For this review, take the finished solid that the model builds, in its own axes (mm). Coordinates: 2 decimals unless noted, no trailing zeros. Write each loop counter-clockwise with the first axis right and the second up, starting at its lowest first coordinate (ties: lowest second). Pieces come first, ordered by that corner, then holes. Notation, with made-up numbers: M 55,36 L 66,36 A16 ccw 66,46 Z; hole C 47.5,54 d4. An arc over 180 degrees is marked long. One line per question, with ' | ' between items.
from build123d import *

# Parameters (mm, degrees)
F0_W     = 240
F0_H     = 55.88
F1_DEPTH = 5


with BuildPart() as f1:
    # F0 (on Top) → F1 (new body)
    with BuildSketch(Plane.XY):
        with Locations((-1.303092, 10.622495)):
            Rectangle(F0_W, F0_H)
        Polygon((-77.501602, 1.566828), (-77.501602, 18.42894), (-73.263034, 18.42894), (-73.263034, 5.436821), (-66.813052, 5.436821), (-66.813052, 1.566828), align=None, mode=Mode.SUBTRACT)
        Polygon((-65.523051, 1.566828), (-65.523051, 18.42894), (-53.171746, 18.42894), (-53.171746, 14.558948), (-61.376628, 14.558948), (-61.376628, 11.610381), (-53.63664, 11.610381), (-53.63664, 8.016816), (-61.284486, 8.016816), (-61.284486, 5.436821), (-52.623071, 5.436821), (-52.623071, 1.566828), align=None, mode=Mode.SUBTRACT)
        Polygon((-46.633799, 1.566828), (-52.623071, 18.42894), (-48.753079, 18.42894), (-44.975229, 7.187532), (-40.736664, 18.42894), (-36.682386, 18.42894), (-43.408804, 1.566828), align=None, mode=Mode.SUBTRACT)
        Polygon((-36.069706, 1.566828), (-36.069706, 18.42894), (-23.595029, 18.42894), (-23.595029, 14.341751), (-32.273065, 14.341751), (-32.273065, 11.978536), (-24.56356, 11.978536), (-24.56356, 7.833225), (-31.885654, 7.833225), (-31.885654, 5.436821), (-23.517547, 5.436821), (-23.517547, 1.566828), align=None, mode=Mode.SUBTRACT)
        Polygon((-22.122035, 1.566828), (-22.122035, 18.42894), (-16.931558, 18.42894), (-16.931558, 5.461609), (-10.812703, 5.461609), (-10.812703, 1.566828), align=None, mode=Mode.SUBTRACT)
        with BuildLine():
            Line((0, 1.486314), (0, 5.613023))
            ThreePointArc((0, 5.613023), (-1.939251, 14.918573), (-3.923162, 5.622442))
            Line((-3.923162, 5.622442), (-3.923162, 1.491197))
            ThreePointArc((-3.923162, 1.491197), (-1.939969, 18.855408), (0, 1.486314))
        make_face(mode=Mode.SUBTRACT)
        Polygon((12.757826, 1.425337), (7.98934, 1.425337), (7.98934, 18.42894), (12.757826, 18.42894), (19.847259, 7.966181), (19.847259, 18.42894), (23.944732, 18.348456), (23.944732, 1.425337), (19.847259, 1.425337), (12.757826, 11.888096), align=None, mode=Mode.SUBTRACT)
        Polygon((26.369521, 1.566828), (26.369521, 18.42894), (38.351353, 18.42894), (38.351353, 14.247308), (30.56819, 14.247308), (30.56819, 12.04724), (38.016446, 12.04724), (38.016446, 7.966181), (30.505024, 7.966181), (30.505024, 5.552883), (39.282415, 5.552883), (39.282415, 1.566828), align=None, mode=Mode.SUBTRACT)
        Polygon((39.282415, 14.247308), (39.282415, 18.42894), (52.912835, 18.42894), (52.912835, 14.247308), (48.958834, 14.247308), (48.958834, 1.566828), (43.528017, 1.566828), (43.528017, 14.247308), align=None, mode=Mode.SUBTRACT)
        Polygon((54.121282, 1.566828), (54.121282, 18.42894), (66.235885, 18.42894), (66.235885, 13.642738), (58.677584, 13.642738), (58.677584, 12.04724), (65.13413, 12.04724), (65.13413, 7.809057), (58.656581, 7.809057), (58.656581, 6.543087), (66.210203, 6.543087), (66.210203, 1.566828), align=None, mode=Mode.SUBTRACT)
        with BuildLine():
            ThreePointArc((81.330004, 16.427406), (81.502994, 13.470076), (78.545664, 13.297086))
            ThreePointArc((78.545664, 13.297086), (71.801666, 10.696378), (77.833893, 6.714239))
            ThreePointArc((77.833893, 6.714239), (80.685897, 5.913115), (79.884773, 3.061112))
            ThreePointArc((79.884773, 3.061112), (67.636498, 11.146737), (81.330004, 16.427406))
        make_face(mode=Mode.SUBTRACT)
        Polygon((83.697356, 1.566828), (83.697356, 18.42894), (88.816062, 18.42894), (88.816062, 12.015753), (93.332559, 12.015753), (93.332559, 18.42894), (98.752365, 18.42894), (98.752365, 1.566828), (93.332559, 1.566828), (93.332559, 7.699986), (88.816062, 7.699986), (88.816062, 1.566828), align=None, mode=Mode.SUBTRACT)
        with BuildLine():
            add(Edge.make_bspline(
                [(101.193711, 16.731108), (99.303506, 15.238125), (99.056959, 11.800154), (101.193711, 10.197595)],
                knots=[0, 0, 0, 0, 6.533513, 6.533513, 6.533513, 6.533513], degree=3))
            add(Edge.make_bspline(
                [(101.193711, 16.731108), (103.618093, 19.223979), (108.672321, 19.539012), (111.685678, 16.67632)],
                knots=[0, 0, 0, 0, 10.49211, 10.49211, 10.49211, 10.49211], degree=3))
            add(Edge.make_bspline(
                [(111.685678, 16.67632), (113.683753, 14.726316), (111.273028, 11.843219), (108.797148, 13.618685)],
                knots=[0, 0, 0, 0, 4.206274, 4.206274, 4.206274, 4.206274], degree=3))
            add(Edge.make_bspline(
                [(108.797148, 13.618685), (107.428901, 14.775181), (105.71859, 15.345286), (105.311371, 14.465697)],
                knots=[0, 0, 0, 0, 3.587209, 3.587209, 3.587209, 3.587209], degree=3))
            add(Edge.make_bspline(
                [(105.311371, 14.465697), (104.073435, 12.592498), (108.808008, 12.174423), (110.556327, 11.028785)],
                knots=[0, 0, 0, 0, 6.270719, 6.270719, 6.270719, 6.270719], degree=3))
            add(Edge.make_bspline(
                [(112.592414, 3.617435), (113.781482, 5.115994), (114.253856, 9.823423), (110.556327, 11.028785)],
                knots=[0, 0, 0, 0, 7.685946, 7.685946, 7.685946, 7.685946], degree=3))
            add(Edge.make_bspline(
                [(100.31075, 3.552281), (104.203738, 0.392276), (110.035092, 0.441142), (112.592414, 3.617435)],
                knots=[0, 0, 0, 0, 12.281837, 12.281837, 12.281837, 12.281837], degree=3))
            add(Edge.make_bspline(
                [(100.31075, 3.552281), (98.51899, 5.230014), (99.903531, 8.911257), (103.47075, 7.51043)],
                knots=[0, 0, 0, 0, 5.064834, 5.064834, 5.064834, 5.064834], degree=3))
            Line((103.47075, 7.51043), (106.353849, 5.588366))
            add(Edge.make_bspline(
                [(107.494056, 7.787338), (110.067666, 7.738471), (108.634263, 4.122384), (106.353849, 5.588366)],
                knots=[0, 0, 0, 0, 2.477004, 2.477004, 2.477004, 2.477004], degree=3))
            add(Edge.make_bspline(
                [(101.193711, 10.197595), (103.193842, 8.732081), (105.327658, 7.803626), (107.494056, 7.787338)],
                knots=[0, 0, 0, 0, 6.745642, 6.745642, 6.745642, 6.745642], degree=3))
        make_face(mode=Mode.SUBTRACT)
        Polygon((-111.039914, 2.497631), (-111.039914, 19.864045), (-104.65432, 19.864045), (-104.65432, 8.465471), (-100.35748, 8.465471), (-100.35748, 2.497631), align=None, mode=Mode.SUBTRACT)
        Polygon((-91.584757, 19.864045), (-91.584757, 2.497631), (-98.089702, 2.497631), (-98.089702, 13.239743), (-102.923647, 13.239743), (-99.581659, 19.864045), align=None, mode=Mode.SUBTRACT)
    extrude(amount=F1_DEPTH)


solid = f1.part
1) We need section B-B on z = 0.8. State how many separate pieces and enclosed holes the cut face has, then the cut area to 3 significant figures.
Responses:
separate pieces: 1 | enclosed holes: 15 | area: 11,200 mm^2
2) We need section A-A on x = 35. State the section outline as (y, z) points, then the cut area to 3 significant figures.
Responses:
outline: M -17.32,0 L 1.57,0 L 1.57,5 L -17.32,5 Z; M 5.55,0 L 7.97,0 L 7.97,5 L 5.55,5 Z; M 12.05,0 L 14.25,0 L 14.25,5 L 12.05,5 Z; M 18.43,0 L 38.56,0 L 38.56,5 L 18.43,5 Z | area: 218 mm^2
3) To check wall thickness, follow line 1 along Y through (x, z) = (37, 3.5); line 2 along Y through (x, z) = (63, 0.75); line 3 along Y through (x, z) = (-107, 0.4). State the ranges of each line that lie inside material, in increasing order. Write a range as [from, to].
Responses:
line 1: [-17.32, 1.57], [5.55, 7.97], [12.05, 14.25], [18.43, 38.56] | line 2: [-17.32, 1.57], [6.54, 7.81], [12.05, 13.64], [18.43, 38.56] | line 3: [-17.32, 2.5], [19.86, 38.56]
